Input: part model. Units: mm. Frame: model coordinates. Give positions to 0.01 mm unless a question says otherwise; leave off trailing zeros. Loops run counter-clockwise (first coordinate to the right, second up) from the corner with the lowest first, then second, coordinate; pieces in that order, holes last. Notation, with made-up numbers: (74.5, 19) - (109.5, 19) arc R27 cw to (109.5, 38) - close; hole circle Ø9 at (-31.75, -26.75). An arc over 180 degrees is marked (long way). Answer as a JSON object with one key per item and string values. Group by question number.
(1) Material intervals for L1, parallel to Y at x = 42, z = 1.3; L2, parallel to Y at x = 44.5, z = 0.55; L3, parallel to Y at x = 6, z = 0.95, sorted ascending.
(2) Section query C-C (z = 0.6). Count the separate pieces of the cut face and the enclosed holes in it, plus the area to 3 significant figures.
(3) Section query B-B (y = 20). Return loops of the section in (x, z).
(4) Section query A-A (x = 116). Return loops of the section in (y, z).
(5) Pin query (flat end, axial travel): P1, Ø2, axis at x = 70, y = 76.5, coming from the -Z side; P2, Ø0.6, axis at y = 29.5, z = 1.5, coming from the -X side; P3, Ø1, axis at x = 88.5, z = 1, coming from the +Y side; P4, Ø1, axis at x = 87.5, z = 1, coming from the -Y side. Return the tip coordinate at first contact, or that it passes through.
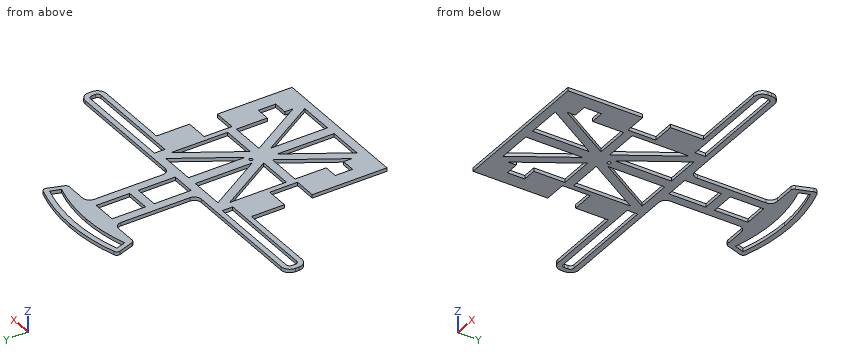
Autodesk Inventor part; units mm, degrees
ref_plane "YZ Plane" through (0, 0, 0) normal (1, 0, 0) x (0, 1, 0)
ref_plane "XZ Plane" through (0, 0, 0) normal (0, 1, 0) x (-1, 0, 0)
ref_plane "XY Plane" through (0, 0, 0) normal (0, 0, 1) x (1, 0, 0)
sketch "Sketch1" plane through (0, 0, 0) normal (0, 0, 1) x (1, 0, 0)
  line L0 (0, 0) -> (42, 0)
  line L1 (42, 0) -> (42, 90)
  line L2 (42, 90) -> (0, 90)
  line L3 (0, 90) -> (0, 0)
  line L4 (0, 90) -> (16, 90)
  line L5 (16, 90) -> (16, 0)
  line L6 (16, 0) -> (0, 0)
  line L7 (0, 0) -> (0, 90)
  line L8 (16, 90) -> (42, 90)
  line L9 (42, 90) -> (42, 85)
  line L10 (42, 85) -> (16, 85)
  line L11 (16, 85) -> (16, 90)
  line L12 (16, 0) -> (42, 0)
  line L13 (42, 0) -> (42, 5)
  line L14 (42, 5) -> (16, 5)
  line L15 (16, 5) -> (16, 0)
  line L16 (16, 47.5) -> (42, 47.5)
  line L17 (42, 47.5) -> (42, 42.5)
  line L18 (42, 42.5) -> (16, 42.5)
  line L19 (16, 42.5) -> (16, 47.5)
  line L20 (0, 90) -> (-44.5, 90)
  line L21 (-49.5, 85) -> (-49.5, 83)
  line L22 (-44.5, 78) -> (0, 78)
  line L23 (0, 78) -> (0, 90)
  arc A0 (-44.5, 90) -> (-49.5, 85) centre (-44.5, 85) ccw
  arc A1 (-49.5, 83) -> (-44.5, 78) centre (-44.5, 83) ccw
  line L24 (-44.5, 87) -> (-3, 87)
  line L25 (-3, 87) -> (-3, 81)
  line L26 (-3, 81) -> (-44.5, 81)
  arc A2 (-46.5, 83) -> (-44.5, 81) centre (-44.5, 83) ccw
  line L27 (-46.5, 83) -> (-46.5, 85)
  arc A3 (-44.5, 87) -> (-46.5, 85) centre (-44.5, 85) ccw
  line L28 (-3, 87) -> (12, 87)
  line L29 (12, 87) -> (12, 81)
  line L30 (12, 81) -> (-3, 81)
  line L31 (-3, 81) -> (-3, 87)
  line L32 (42, 85) -> (39, 85)
  line L33 (39, 85) -> (39, 5)
  line L34 (39, 5) -> (42, 5)
  line L35 (42, 5) -> (42, 85)
  circle A4 centre (42, 51.037) radius 1
  line L36 (16, 85) -> (39, 47.5) construction
  line L37 (39, 42.5) -> (16, 5) construction
  line L38 (18.9328, 85) -> (39, 52.2817)
  line L39 (36.0672, 47.5) -> (16, 80.2183)
  line L40 (36.0672, 42.5) -> (16, 9.7817)
  line L41 (18.9328, 5) -> (39, 37.7183)
  point P0 (16, 45)
  point P1 (16, 45)
  point P2 (-49.5, 78)
  point P3 (-49.5, 90)
  point P4 (27.5, 23.75)
  point P5 (16, 42.5)
  point P6 (0, 78)
  point P7 (42, 50.037)
  point P8 (42, 52.037)
  dimension "d0" = 42
  dimension "d1" = 90
  dimension "d2" = 16
  dimension "d3" = 5
  dimension "d4" = 26
  dimension "d5" = 5
  dimension "d6" = 26
  dimension "d7" = 5
  dimension "d8" = 49.5
  dimension "d9" = 12
  dimension "d10" = 5
  dimension "d11" = 3
  dimension "d12" = 15
  dimension "d13" = 6
  dimension "d14" = 3
  dimension "d17" = 2
  dimension "d19" = 38.963
  dimension "d20" = 2.5
  dimension "d21" = 2.5
  dimension "d22" = 2.5
  dimension "d23" = 2.5
extrude "Extrusion1" add sketch "Sketch1" along normal blind 2 contours L3 L30 L29 L28 L2 L5 L0 | L5 L14 L1 L0 | L22 A1 L21 A0 L20 L3 L28 L24 A3 L27 A2 L26 L30 | L5 L40 L18 L33 L41 L14 | L14 L33 L18 L1 | L18 L33 L16 L1 | L5 L16 L33 L18 | L16 L33 L10 L1 A4 | L2 L1 L10 L5 | L16 L39 L5 L10 L38 L33
sketch "Sketch2" plane through (0, 0, 2) normal (0, 0, 1) x (1, 0, 0)
  arc A0 (42, 52.037) -> (42, 50.037) centre (42, 51.037) ccw
  circle A1 centre (42, 51.037) radius 104 construction
  circle A2 centre (42, 51.037) radius 101 construction
  circle A3 centre (42, 51.037) radius 95 construction
  circle A4 centre (42, 51.037) radius 93 construction
  line L0 (42, 90) -> (-44.5, 90)
  line L1 (42, 90) -> (42, -52.963)
  line L2 (42, 155.037) -> (42, 90)
  line L3 (42, 51.037) -> (8.6562, 149.5469) construction
  line L4 (42, 51.037) -> (146, 51.037) construction
  line L5 (42, 51.037) -> (13.2923, 139.4953) construction
  line L6 (42, 51.037) -> (135, 51.037) construction
  line L7 (42, 51.037) -> (12.3019, 147.5721) construction
  line L8 (42, 51.037) -> (143, 51.037) construction
  line L9 (12.3019, 147.5721) -> (14.0662, 141.8373)
  arc A5 (42, 152.037) -> (12.3019, 147.5721) centre (42, 51.037) ccw
  arc A6 (42, 146.037) -> (14.0662, 141.8373) centre (42, 51.037) ccw
  line L10 (14.0662, 141.8373) -> (16.0662, 141.8373) construction
  line L11 (13.2923, 139.4953) -> (13.2923, 137.4953) construction
  line L12 (9.3038, 147.6339) -> (12.2756, 138.8541)
  arc A7 (42, 155.037) -> (10.5942, 150.1817) centre (42, 51.037) ccw
  line L13 (42, 90) -> (30, 90)
  line L14 (30, 94) -> (30, 133.4953)
  line L15 (30, 137.4953) -> (42, 137.4953)
  line L16 (42, 137.4953) -> (42, 90)
  line L17 (14.17, 137.4953) -> (26, 137.4953)
  line L18 (30, 137.4953) -> (35, 137.4953)
  line L19 (35, 137.4953) -> (35, 90)
  line L20 (35, 90) -> (30, 90)
  line L21 (30, 90) -> (30, 137.4953)
  line L22 (35, 137.4953) -> (42, 137.4953)
  line L23 (42, 137.4953) -> (42, 135.4953)
  line L24 (42, 135.4953) -> (35, 135.4953)
  line L25 (35, 135.4953) -> (35, 137.4953)
  line L26 (35, 116.2476) -> (42, 116.2476)
  line L27 (42, 116.2476) -> (42, 111.2476)
  line L28 (42, 111.2476) -> (35, 111.2476)
  line L29 (35, 111.2476) -> (35, 116.2476)
  arc A8 (10.5942, 150.1817) -> (9.3038, 147.6339) centre (11.1982, 148.2751) ccw
  arc A9 (12.2756, 138.8541) -> (14.17, 137.4953) centre (14.17, 139.4953) ccw
  line L30 (26, 90) -> (26, 90)
  arc A10 (26, 90) -> (30, 94) centre (26, 94) ccw
  arc A11 (30, 133.4953) -> (26, 137.4953) centre (26, 133.4953) ccw
  point P0 (0, 0)
  point P1 (12.7355, 137.4953)
  point P2 (35, 113.7476)
  point P3 (35, 113.7476)
  point P4 (42, 152.037)
  dimension "d27" = 202
  dimension "d29" = 186
  dimension "d26" = 208
  dimension "d28" = 190
  dimension "d30" = 108.7
  dimension "d31" = 107.98
  dimension "d32" = 101
  dimension "d33" = 107.1
  dimension "d36" = 2
  dimension "d37" = 12
  dimension "d38" = 5
  dimension "d39" = 2
  dimension "d40" = 7
  dimension "d41" = 5
  dimension "d42" = 2
  dimension "d43" = 2
  dimension "d44" = 4
  dimension "d45" = 4
extrude "Extrusion2" add sketch "Sketch2" against normal blind 2 contours L0 L21 L14 L15 L19 | L28 L19 L26 L2 | L0 A10 L21 | L24 L19 L15 L2 | A11 L17 A9 L12 A8 A7 L2 A5 L9 A6 L15 L21
sketch "Sketch3" plane through (0, 0, 2) normal (0, 0, 1) x (1, 0, 0)
  line L0 (0, 59.037) -> (13, 59.037)
  line L1 (13, 59.037) -> (13, 43.037)
  line L2 (13, 43.037) -> (0, 43.037)
  line L3 (0, 43.037) -> (0, 59.037)
  line L4 (12, 81) -> (-44.5, 81)
  line L5 (0, 78) -> (0, 0)
  line L6 (16, 9.7817) -> (16, 42.5)
  line L7 (16, 24.589) -> (8, 24.589)
  line L8 (8, 24.589) -> (8, 14.589)
  line L9 (8, 14.589) -> (16, 14.589)
  line L10 (16, 14.589) -> (16, 24.589)
  line L11 (0, 0) -> (42, 0)
  line L12 (26, 90) -> (-44.5, 90)
  point P0 (0, 51.037)
  point P1 (16, 19.589)
  dimension "d48" = 13
  dimension "d49" = 16
  dimension "d51" = 0
  dimension "d52" = 8
  dimension "d53" = 10
  dimension "d54" = 19.589
  dimension "d55" = 38.963
extrude "Extrusion3" cut sketch "Sketch3" against normal through all
mirror "Mirror2" about plane through (42, 52.037, 0) normal (1, 0, 0)
properties part number "StructureV2Laser"
Recorded:
{
 "1": {"L1": "y = 0 to 50.04, 52.04 to 90, 111.25 to 116.25, 135.5 to 146.04, 152.04 to 155.04", "L2": "y = 0 to 90, 111.25 to 116.25, 135.5 to 146, 152.01 to 155.01", "L3": "y = 0 to 43.04, 59.04 to 81, 87 to 90"},
 "2": {"separate pieces": "1", "enclosed holes": "14", "area": "6,060 mm^2"},
 "3": {"outline": "(0, 0) - (8, 0) - (8, 2) - (0, 2) - close; (22.27, 0) - (28.13, 0) - (28.13, 2) - (22.27, 2) - close; (39, 0) - (45, 0) - (45, 2) - (39, 2) - close; (55.87, 0) - (61.73, 0) - (61.73, 2) - (55.87, 2) - close; (76, 0) - (84, 0) - (84, 2) - (76, 2) - close"},
 "4": {"outline": "(78, 0) - (81, 0) - (81, 2) - (78, 2) - close; (87, 0) - (90, 0) - (90, 2) - (87, 2) - close"},
 "5": {"P1": "stops at z = 0", "P2": "stops at x = 0", "P3": "stops at y = 90", "P4": "stops at y = 78"}
}
